```python
from build123d import *

# Parameters (mm, degrees)
SKETCH1_R           = 2.25
BOSS_EXTRUDE1_DEPTH = 45
SKETCH2_R           = 4
BOSS_EXTRUDE2_DEPTH = 4
FILLET1_R           = 1.5


with BuildPart() as part:
    # Sketch1 → Boss-Extrude1 (new body)
    with BuildSketch(Plane.XY):
        with Locations(Location((0, 0, 0), (0, 0, 180))):
            Circle(SKETCH1_R)
    extrude(amount=BOSS_EXTRUDE1_DEPTH)

    # Sketch2 → Boss-Extrude2 (add)
    with BuildSketch(Plane.XY.offset(45)):
        Circle(SKETCH2_R)
    extrude(amount=BOSS_EXTRUDE2_DEPTH)

    # Fillet1
    fillet1_edges = [part.edges().sort_by_distance(p)[0] for p in [
        (-4, 0, 45),
        (-4, 0, 49),
    ]]
    fillet(fillet1_edges, radius=FILLET1_R)


solid = part.part
```
Input: part model. Units: mm. Frame: model coordinates. A direction names the side the tool comes from. Round coordinates to 2 decimals unless told otherwise and drop trailing zeros. Loops run counter-clockwise (first coordinate to the right, second up) from the corner with the lowest first, then second, coordinate; pieces in that order, holes last.
1) Set-up query: faces 1 (the flat face through (0, 0, 49)), 2 (the cylindrical face through (1.66, -1.52, 22.18)). Return all of +Z, -Z, +X, -X, +Y, -Y with unobstructed straight access to the full face (end or side cutting, diameter ignored); none if empty.
Ans:
face 1: +Z, +X, -X, +Y, -Y
face 2: -Z
2) Pin query (flat end, axial travel): pin 1 (1.5 mm diameter, centred on x = 0.5, z = 31.5, fed in from +Y); pin 2 (1.5 mm diameter, centred on x = -0.5, y = 1.5, fed in from -Z); pin 3 (4 mm diameter, centred on y = 0.5, z = 10.5, fed in from -X). Return the tip coordinate at first contact, or that it passes through.
Ans:
pin 1: stops at y = 2.25
pin 2: stops at z = 0
pin 3: stops at x = -2.25
3) Section query A-A on x = 0. Return the cut outline in (y, z).
Ans:
outline: (-4, 46.5) arc R1.5 ccw to (-2.5, 45) - (-2.25, 45) - (-2.25, 0) - (2.25, 0) - (2.25, 45) - (2.5, 45) arc R1.5 ccw to (4, 46.5) - (4, 47.5) arc R1.5 ccw to (2.5, 49) - (-2.5, 49) arc R1.5 ccw to (-4, 47.5) - close
4) Material intervals for line 1 (Z direction, x = -2.25, y = 0.5); line 2 (Y direction, x = -2, z = 20.5); line 3 (Z direction, x = 2.75, y = 1.75), sorted ascending.
Ans:
line 1: z = 45 to 49
line 2: y = -1.03 to 1.03
line 3: z = 45.21 to 48.79
5) Section query C-C on z = 4.5. Return the cut outline in (x, y), plus the area to 3 significant figures.
Ans:
outline: circle Ø4.5 at (0, 0)
area: 15.9 mm2
